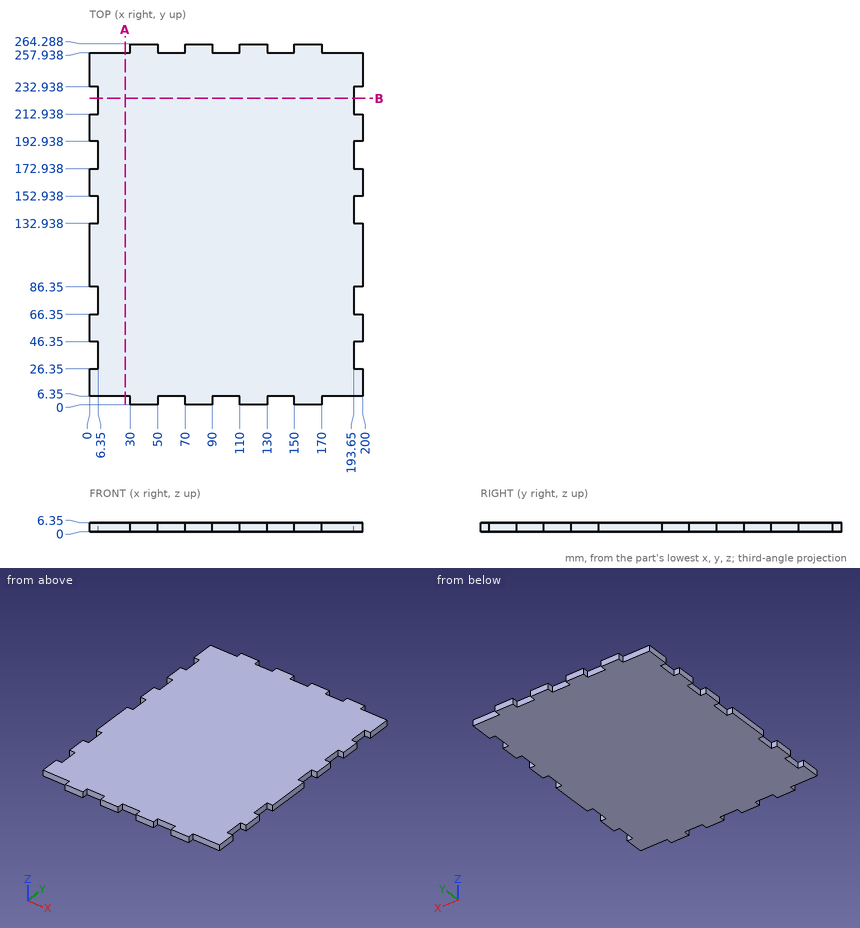
Part print with two shaded views. Sizes in mm from the minimum x, y, z corner. Round coordinates to 2 decimals unless told otherwise and drop trailing zeros. Order: outer loops, then holes, each group sorted by start corner. A loop starts at its lowest first (then second) coordinate and runs counter-clockwise, first axis right, second up. Notation, with made-up numbers: M -27,39 L -4,39 A6 ccw -4,47 Z; hole C -23.5,84 d1. An arc over 180 degrees is marked long. Put each result on its own line as item: value. Start each with the question number.
1. Slice it at A-A on x = 26. List the corners of the cut face in (y, z).
2. Drop flat-ended pins along their axis: pin 1 (1.9 mm diameter, centred on y = 260.5, z = 2.5, fed in from +X); pin 2 (1.9 mm diameter, centred on x = 104, z = 2, fed in from +Y); pin 3 (1.9 mm diameter, centred on x = 2.5, z = 2.5, fed in from -Y). Give the stop position or say it passes through.
3. Slice it at B-B on y = 224.5. List the corners of the cut face in (x, z).
4. Drill centre lines: probe 1 along X at (y, z) = (72, 4.25); probe 2 along Y at (x, z) = (188, 0.5). Where is each one in solid material? Low to high. Write a range as [from, to].
Findings:
1. outline: M 6.35,0 L 257.94,0 L 257.94,6.35 L 6.35,6.35 Z
2. pin 1: x = 170
2. pin 2: y = 257.94
2. pin 3: y = 6.35
3. outline: M 6.35,0 L 193.65,0 L 193.65,6.35 L 6.35,6.35 Z
4. probe 1: [6.35, 193.65]
4. probe 2: [6.35, 257.94]
